Check sheet for the modelled part. Datum: model origin and axes. Units: mm. Round coordinates to 2 decimals unless told otherwise and drop trailing zeros. Order: outer loops, then holes, each group sorted by start corner. A loop starts at its lowest first (then second) coordinate and runs counter-clockwise, first axis right, second up.
```python
from build123d import *

# Parameters (mm, degrees)
SKETCH1_R           = 26.5
BOSS_EXTRUDE1_DEPTH = 5
SKETCH2_R           = 25.25
BOSS_EXTRUDE2_DEPTH = 10
SKETCH3_R           = 26.5
BOSS_EXTRUDE3_DEPTH = 5
SKETCH4_R           = 5
CUT_EXTRUDE1_DEPTH  = 43.479406776
CUT_EXTRUDE2_DEPTH  = 43.479406776
FILLET1_R           = 2


with BuildPart() as part:
    # Sketch1 → Boss-Extrude1 (new body)
    with BuildSketch(Plane.XY):
        Circle(SKETCH1_R)
    extrude(amount=BOSS_EXTRUDE1_DEPTH)

    # Sketch2 → Boss-Extrude2 (add)
    with BuildSketch(Plane.XY.offset(5)):
        Circle(SKETCH2_R)
    extrude(amount=BOSS_EXTRUDE2_DEPTH)

    # Sketch3 → Boss-Extrude3 (add)
    with BuildSketch(Plane.XY.offset(15)):
        Circle(SKETCH3_R)
    extrude(amount=BOSS_EXTRUDE3_DEPTH)

    # Sketch4 → Cut-Extrude1 (cut, through all)
    with BuildSketch(Plane.XY.offset(20)):
        Circle(SKETCH4_R)
    extrude(amount=-CUT_EXTRUDE1_DEPTH, mode=Mode.SUBTRACT)

    # Sketch6 → Cut-Extrude2 (cut, through all)
    with BuildSketch(Plane.XY.offset(20)):
        with BuildLine():
            ThreePointArc((-10, 0), (-8.660254038, 5), (-5, 8.660254038))
            Line((-5, 8.660254038), (-5, 19.623009453))
            ThreePointArc((-5, 19.623009453), (-17.537014427, 10.125), (-19.494024685, -5.481377708))
            Line((-19.494024685, -5.481377708), (-10, 0))
        make_face()
        with BuildLine():
            Line((14.494024685, -14.141631746), (5, -8.660254038))
            ThreePointArc((5, -8.660254038), (0, -10), (-5, -8.660254038))
            Line((-5, -8.660254038), (-14.494024685, -14.141631746))
            ThreePointArc((-14.494024685, -14.141631746), (0, -20.25), (14.494024685, -14.141631746))
        make_face()
        with BuildLine():
            Line((5, 19.623009453), (5, 8.660254038))
            ThreePointArc((5, 8.660254038), (8.660254038, 5), (10, 0))
            Line((10, 0), (19.494024685, -5.481377708))
            ThreePointArc((19.494024685, -5.481377708), (20.0601159, -2.766631537), (20.25, 0))
            ThreePointArc((20.25, 0), (15.989254204, 12.426031144), (5, 19.623009453))
        make_face()
    extrude(amount=-CUT_EXTRUDE2_DEPTH, mode=Mode.SUBTRACT)

    # Fillet1
    fillet1_edges = [part.edges().sort_by_distance(p)[0] for p in [
        (10, 0, 10),
        (5, 8.660254038, 10),
        (5, 19.623009453, 10),
        (19.494024685, -5.481377708, 10),
        (-5, -8.660254038, 10),
        (5, -8.660254038, 10),
        (14.494024685, -14.141631746, 10),
        (-14.494024685, -14.141631746, 10),
        (-5, 8.660254038, 10),
        (-10, 0, 10),
        (-19.494024685, -5.481377708, 10),
        (-5, 19.623009453, 10),
    ]]
    fillet(fillet1_edges, radius=FILLET1_R)


solid = part.part
```
Item 1: Scan lines: line 1 along X through (y, z) = (6, 10); line 2 along Y through (x, z) = (-11, 4.75); line 3 along Y through (x, z) = (9, 10). Record each from-to range of solid material in increasing order.
Answer:
line 1: x = -24.53 to -19.34, -8 to 8, 19.34 to 24.53
line 2: y = -24.11 to -17, -12.12 to -0.58, 17 to 24.11
line 3: y = -23.59 to -18.14, -10.97 to 4.36, 18.14 to 23.59
Item 2: Sectioned sample at C-C (x = 0). Record the cut outline in (y, z), and give its area (3 significant figures).
Answer:
outline: (-26.5, 0) - (-20.25, 0) - (-20.25, 20) - (-26.5, 20) - (-26.5, 15) - (-25.25, 15) - (-25.25, 5) - (-26.5, 5) - close; (-10, 0) - (-5, 0) - (-5, 20) - (-10, 20) - close; (5, 0) - (26.5, 0) - (26.5, 5) - (25.25, 5) - (25.25, 15) - (26.5, 15) - (26.5, 20) - (5, 20) - close
area: 630 mm2
Item 3: Sectioned sample at A-A (z = 18). Record the cut outline in (x, y).
Answer:
outline: circle Ø53 at (0, 0); hole (-20.08, -2.62) arc R2 ccw to (-17.1, -4.1) - (-10.94, -0.54) arc R2 ccw to (-9.95, 0.99) arc R10 cw to (-5.83, 8.12) arc R2 ccw to (-5, 9.75) - (-5, 16.85) arc R2 ccw to (-7.77, 18.7) arc R20.25 ccw to start; hole (-12.31, -16.08) arc R20.25 ccw to (12.31, -16.08) arc R2 ccw to (12.1, -12.76) - (5.94, -9.2) arc R2 ccw to (4.12, -9.11) arc R10 cw to (-4.12, -9.11) arc R2 ccw to (-5.94, -9.2) - (-12.1, -12.76) arc R2 ccw to start; hole circle Ø10 at (0, 0); hole (5, 9.75) arc R2 ccw to (5.83, 8.12) arc R10 cw to (9.95, 0.99) arc R2 ccw to (10.94, -0.54) - (17.1, -4.1) arc R2 ccw to (20.08, -2.62) arc R20.25 ccw to (7.77, 18.7) arc R2 ccw to (5, 16.85) - close
Item 4: Sectioned sample at B-B (y = 16). Record the cut outline in (x, z), and give its area (3 significant figures).
Answer:
outline: (-21.12, 0) - (-12.41, 0) - (-12.41, 20) - (-21.12, 20) - (-21.12, 15) - (-19.53, 15) - (-19.53, 5) - (-21.12, 5) - close; (-5, 0) - (5, 0) - (5, 20) - (-5, 20) - close; (12.41, 0) - (21.12, 0) - (21.12, 5) - (19.53, 5) - (19.53, 15) - (21.12, 15) - (21.12, 20) - (12.41, 20) - close
area: 517 mm2
Item 5: Go/stop test with flat-tipped pins: P1, Ø3.5, axis at y = 12, z = 13, coming from the -X side; P2, Ø2, axis at x = -8, z = 10, coming from the -Y side; P3, Ø6, axis at x = 6, z = 15.5, coming from the -Y side. Record where each tip stops, or that it passes through.
Answer:
P1: stops at x = -23.08
P2: stops at y = -24.26
P3: stops at y = -26.33
Item 6: Sectioned sample at D-D (y = -17). Record the cut outline in (x, z), and give its area (3 significant figures).
Answer:
outline: (-20.33, 0) - (-11, 0) - (-11, 20) - (-20.33, 20) - (-20.33, 15) - (-18.67, 15) - (-18.67, 5) - (-20.33, 5) - close; (11, 0) - (20.33, 0) - (20.33, 5) - (18.67, 5) - (18.67, 15) - (20.33, 15) - (20.33, 20) - (11, 20) - close
area: 340 mm2
Item 7: Release check for a two-part mould opening along Y. For faces 1 (the cylindrical face through (14.246, 22.345, 2.465)), 2 (the flat face through (0, -6, 20)), 3 (the cylindrical face through (-5.867, 18.502, 9.86)) record: released by +Y, released by -Y, zero draft, split by the parting line, or undercut.
Answer:
face 1: split by the parting line
face 2: zero draft
face 3: undercut
